Could you check a few things on this model? Use its own coordinates, in mm. Face numbers are marked on the shaded views. A direction names the side the tool comes from. Coordinates: 2 decimals unless noted, no trailing zeros. Write each loop counter-clockwise with the first axis right and the second up, starting at its lowest first coordinate (ties: lowest second). Pieces come first, ordered by that corner, then holes. Notation, with made-up numbers: (-35.75, 72.5) - (-5.75, 72.5) arc R27 cw to (-5.75, 102.5) - close; hole circle Ø3 at (-28, -16.5). An arc over 180 degrees is marked (long way). Write item = value, one per line. Start each with the question number.
Autodesk Inventor part; units mm, degrees
ref_plane "YZ Plane" through (0, 0, 0) normal (1, 0, 0) x (0, 1, 0)
ref_plane "XZ Plane" through (0, 0, 0) normal (0, 1, 0) x (-1, 0, 0)
ref_plane "XY Plane" through (0, 0, 0) normal (0, 0, 1) x (1, 0, 0)
sketch "Sketch1" plane through (0, 0, 0) normal (1, 0, 0) x (0, 1, 0)
  circle A0 centre (0, 0) radius 3
  dimension "d0" = 6
extrude "Extrusion1" add sketch "Sketch1" along normal blind 20
sketch "Sketch2" plane through (20, 0, 0) normal (1, 0, 0) x (0, 0, -1)
  circle A0 centre (0, 0) radius 3
  circle A1 centre (0, 0) radius 1
  dimension "d3" = 2
extrude "Extrusion2" add sketch "Sketch2" along normal blind 3 contours A1
sketch "Sketch3" plane through (20, 0, 0) normal (1, 0, 0) x (0, 0, -1)
  circle A0 centre (0, 0) radius 1
  circle A1 centre (0, 0) radius 3
  line L0 (3, 0) -> (3.1, 0)
  line L1 (3.1, 0) -> (3.1, -1)
  line L2 (3.1, -1) -> (3.1, 1)
  line L3 (3.1, 1) -> (2.8284, 1)
  circle A2 centre (0, 0) radius 3
  line L4 (3.1, -1) -> (2.8284, -1)
  dimension "d6" = 0.1
  dimension "d7" = 2
extrude "Extrusion3" add sketch "Sketch3" against normal up to surface (20 mm away) contours L0 L1 L4 A1 | A1 L3 L2 L0
properties part number "silnik_2"
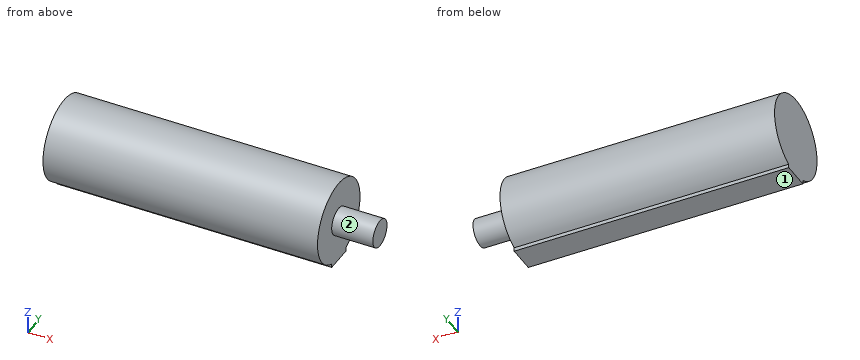
1) Which directions (+Z, -Z, +X, -X, +Y, -Y) give clear straight access to the entire face, cutting with the end or side of a thin tool? Please do the marked faces 1 and 2.
2) Suppose I cut it at D-D on z = -2.5. Please give me the cut outline in (x, y).
3) For P1, Ø1, axis at y = 0, z = 2, coming from the +X side; P2, Ø2, axis at x = 17, y = 2.5, coming from the -Z side; P3, Ø1, axis at x = 5, z = 1, coming from the -Y side, each with a flat end and sliding along its axis, tell me the tip position at first contact or that it passes through.
4) Suppose I cut it at A-A on y = 0. Please give me the cut outline in (x, z).
5) If I drill on probe 1 along X at (y, z) = (1.5, 0); probe 2 along Y at (x, z) = (16.25, 2.5); probe 3 along Z at (x, y) = (19.75, 0.5), over which ranges is the centre line in solid material (lowest first)? Write a range as [from, to].
6) Suppose I cut it at C-C on x = 19. Please give me the cut outline in (y, z).
7) Suppose I cut it at B-B on z = 0. Please give me the cut outline in (x, y), plus the area to 3 significant figures.
Reply:
q1.face_1 = -Z, +X, -X, +Y, -Y
q1.face_2 = +X
q2.outline = (0, -1.66) - (20, -1.66) - (20, 1.66) - (0, 1.66) - close
q3.P1 = 20
q3.P2 = -2.6
q3.P3 = -2.96
q4.outline = (0, -3.1) - (20, -3.1) - (20, -1) - (23, -1) - (23, 1) - (20, 1) - (20, 3) - (0, 3) - close
q5.probe_1 = [0, 20]
q5.probe_2 = [-1.66, 1.66]
q5.probe_3 = [-3.1, 2.96]
q6.outline = (-1, -3.1) - (1, -3.1) - (1, -2.83) arc R3 ccw (long way) to (-1, -2.83) - close
q7.outline = (0, -3) - (20, -3) - (20, -1) - (23, -1) - (23, 1) - (20, 1) - (20, 3) - (0, 3) - close
q7.area = 126 mm^2
